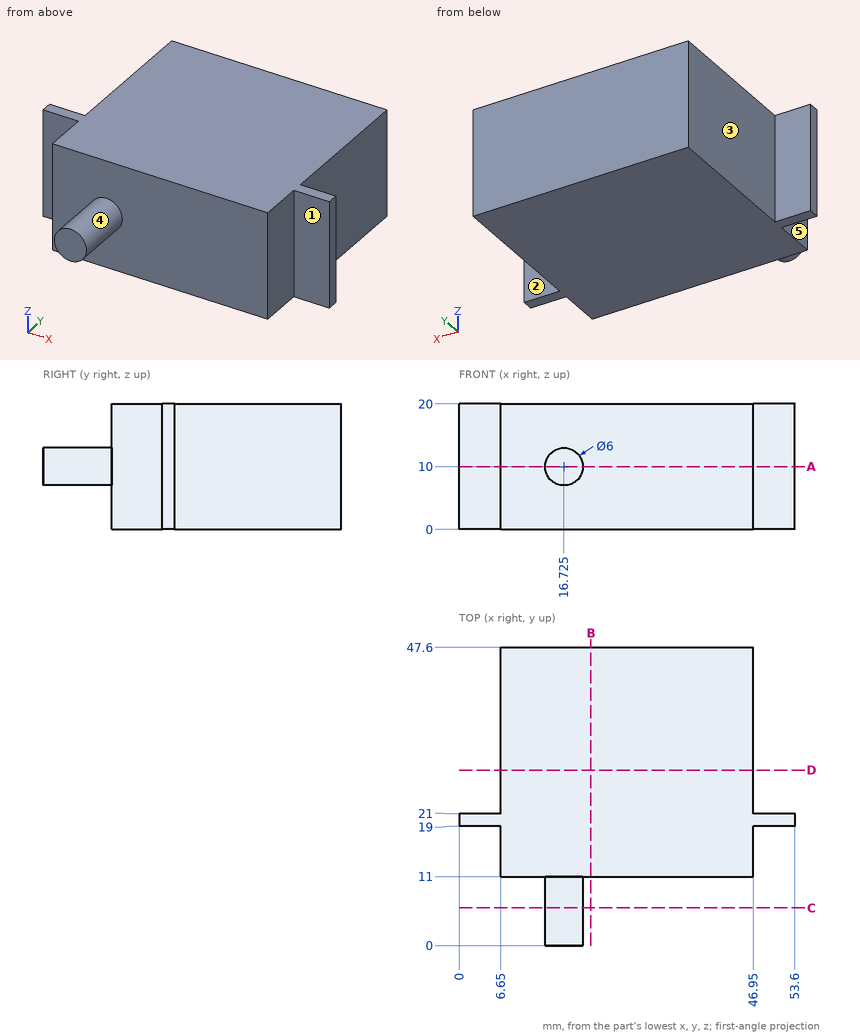
Can you work these out from the drawing? Everything is in mm from the part's minimum corner. A direction names the side the tool comes from. Round coordinates to 2 decimals unless told otherwise and drop trailing zeros. Order: outer loops, then holes, each group sorted by start corner. A loop starts at its lowest first (then second) coordinate and runs counter-clockwise, first axis right, second up. Notation, with made-up numbers: M -19.5,85.5 L 24.5,85.5 A14 ccw 24.5,94.5 Z; hole C 2,-4 d10. An arc over 180 degrees is marked long. Answer as CSV lines item,"result".
Item 1: Imagine slicing it at C-C on y = 6. List the corners of the cut face in (x, z) for me (3 decimals), and give its area (3 significant figures).
From the geometry:
outline,"C 16.725,10 d6"
area,"28.3 mm2"
Item 2: Imagine slicing it at D-D on y = 28. List the corners of the cut face in (x, z) for me.
From the geometry:
outline,"M 6.65,0 L 46.95,0 L 46.95,20 L 6.65,20 Z"
Item 3: Imagine slicing it at A-A on z = 10. List the corners of the cut face in (x, y) for me (3 decimals).
From the geometry:
outline,"M 0,19 L 6.65,19 L 6.65,11 L 13.725,11 L 13.725,0 L 19.725,0 L 19.725,11 L 46.95,11 L 46.95,19 L 53.6,19 L 53.6,21 L 46.95,21 L 46.95,47.6 L 6.65,47.6 L 6.65,21 L 0,21 Z"
Item 4: Which directions (+Z, -Z, +X, -X, +Y, -Y) give clear straight access to the entire face, cutting with the end or side of a thin tool? Please do the marked faces 1, 2, 3, 4 and 5.
From the geometry:
face 1,"+Z, -Z, +X, -Y"
face 2,"+Z, -Z, +X, +Y"
face 3,"+Z, -Z, -X, +Y"
face 4,"-Y"
face 5,"+Z, -Z, -X, -Y"
Item 5: Please list where these lines run through material, in increasing order: L1, parallel to X at y = 13, z = 5.5; L2, parallel to Y at x = 17, z = 16.25. Write a range as [from, to].
From the geometry:
L1,"[6.65, 46.95]"
L2,"[11, 47.6]"
Item 6: For pin 1 (9 mm diameter, centred on y = 13, z = 8, fed in from -X); pin 2 (3.5 mm diameter, centred on x = 3.5, z = 12, fed in from -Y); pin 3 (6 mm diameter, centred on y = 28.5, z = 4, fed in from +X); pin 4 (1.5 mm diameter, centred on x = 11.5, y = 8, fed in from +Z), each with a flat end and sliding along its axis, tell me the tip position at first contact or that it passes through.
From the geometry:
pin 1,"x = 6.65"
pin 2,"y = 19"
pin 3,"x = 46.95"
pin 4,"through"
Item 7: Imagine slicing it at B-B on x = 21. List the corners of the cut face in (y, z) for me, and give its area (3 significant figures).
From the geometry:
outline,"M 11,0 L 47.6,0 L 47.6,20 L 11,20 Z"
area,"732 mm2"
